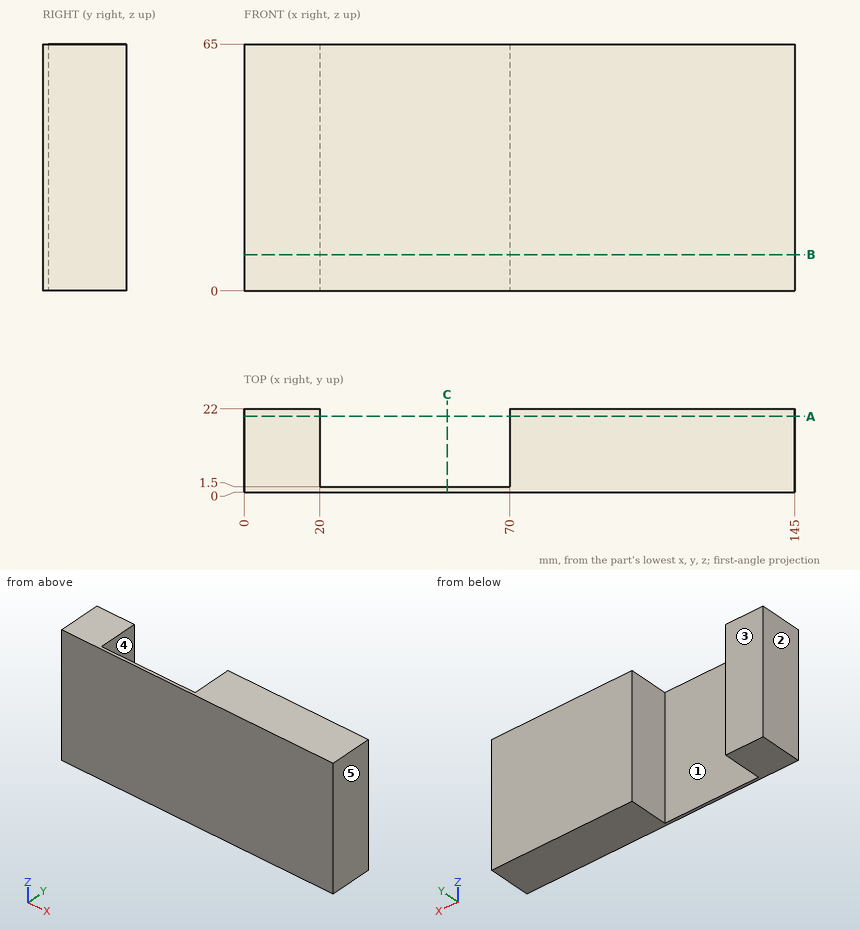
Design review of the part shown in the three views and the two pictorial views. Dimensions are in mm from the part's minimum x, y and z. A direction names the side the tool comes from. Coordinates: 2 decimals unless noted, no trailing zeros. Write each loop counter-clockwise with the first axis right and the second up, starting at its lowest first coordinate (ties: lowest second). Pieces come first, ordered by that corner, then holes.
1) We need section C-C on x = 53.5. State the section outline as (y, z) points, then the cut area to 3 significant figures.
2) We need section B-B on z = 9.5. State the section outline as (x, y) points, then the cut area to 4 significant figures.
3) Clearance check with a flat-ended pin moving along its axis: pin 1 Ø15 at (x, z) = (50, 34) entering from +Y. State where the tip first meets the part, or that it passes through.
4) We need section A-A on y = 20. State the section outline as (x, z) points, then the cut area to 4 significant figures.
5) Machinability: for the marked faces 4 and 5, which of the approach directions +Z, -Z, +X, -X, +Y, -Y give a long, thin tool a straight path to every point of the face, cutting with its end or side? Answer none if there is none.
6) To check wall thickness, follow probe 1 along X at (y, z) = (11, 10); probe 2 along Y at (x, z) = (59, 49). State the ranges of each line that lie inside material, in increasing order.
7) The part is to be moulded in two halves that separate along X. For the marked faces 1, 2 and 3, say which applies: pulls with the +X half, pulls with the -X half, needs draft (parallel to the pull), parting line crosses it, or undercut.
Answer list:
1. outline: (0, 0) - (1.5, 0) - (1.5, 65) - (0, 65) - close
1. area: 97.5 mm2
2. outline: (0, 0) - (145, 0) - (145, 22) - (70, 22) - (70, 1.5) - (20, 1.5) - (20, 22) - (0, 22) - close
2. area: 2,165 mm2
3. pin 1: stops at y = 1.5
4. outline: (0, 0) - (20, 0) - (20, 65) - (0, 65) - close; (70, 0) - (145, 0) - (145, 65) - (70, 65) - close
4. area: 6,175 mm2
5. face 4: +Z, -Z, +Y
5. face 5: +Z, -Z, +X, +Y, -Y
6. probe 1: x = 0 to 20, 70 to 145
6. probe 2: y = 0 to 1.5
7. face 1: undercut
7. face 2: pulls with the -X half
7. face 3: needs draft
